The listing builds one solid part. Answer for the finished solid, in the listing's coordinates (mm). A direction names the side the tool comes from. Round coordinates to 2 decimals unless told otherwise and drop trailing zeros. Loops run counter-clockwise (first coordinate to the right, second up) from the corner with the lowest first, then second, coordinate; pieces in that order, holes last. Notation, with made-up numbers: M 58.5,5.5 L 106.5,5.5 A23 ccw 106.5,43.5 Z; hole C 87.25,27.25 d1. An arc over 180 degrees is marked long. Answer as a JSON object with one key per item and string values.
```python
from build123d import *

# Parameters (mm, degrees)
BOSS_EXTRUDE1_DEPTH = 20
SKETCH2_R           = 2.25
SKETCH2_R_2         = 5.25
CUT_EXTRUDE1_DEPTH  = 40


with BuildPart() as part:
    # Sketch1 → Boss-Extrude1 (new, symmetric)
    with BuildSketch(Plane.XY):
        Polygon((-150, 7.75), (-150, -7.75), (150, -7.75), (150, 7.75), (20, 7.75), (20, 0.25), (-20, 0.25), (-20, 7.75), align=None)
    extrude(amount=BOSS_EXTRUDE1_DEPTH, both=True)

    # Sketch2 → Cut-Extrude1 (cut)
    with BuildSketch(Plane(origin=(0, 0.25, 0), x_dir=(1, 0, 0), z_dir=(0, 1, 0))):
        with Locations(Location((15.015, 15, 0), (0, 0, 270))):
            Circle(SKETCH2_R)
        with Locations(Location((-15.015, 15, 0), (0, 0, 180))):
            Circle(SKETCH2_R)
        with Locations(Location((15.015, -15, 0), (0, 0, 180))):
            Circle(SKETCH2_R)
        with Locations(Location((-15.015, -15, 0), (0, 0, 270))):
            Circle(SKETCH2_R)
        with Locations(Location((0, 0, 0), (0, 0, 270))):
            Circle(SKETCH2_R_2)
    extrude(amount=-CUT_EXTRUDE1_DEPTH, mode=Mode.SUBTRACT)


solid = part.part
```
Item 1: The part is cut by section B-B (x = 0). Give the vertices of the cut face in (y, z).
Values follow:
{"outline": "M -7.75,-20 L 0.25,-20 L 0.25,-5.25 L -7.75,-5.25 Z; M -7.75,5.25 L 0.25,5.25 L 0.25,20 L -7.75,20 Z"}
Item 2: Straight lines are drawn through the part: line 1 (X direction, y = -5.75, z = 15.5); line 2 (X direction, y = 1, z = 9.5); line 3 (X direction, y = -3.75, z = -16.5). For each, find the intervals that lie inside material, in ascending order.
Values follow:
{"line 1": "-150 to -17.21, -12.82 to 12.82, 17.21 to 150", "line 2": "-150 to -20, 20 to 150", "line 3": "-150 to -16.69, -13.34 to 13.34, 16.69 to 150"}
Item 3: The part is cut by section A-A (z = 0). Give the vertices of the cut face in (x, y).
Values follow:
{"outline": "M -150,-7.75 L -5.25,-7.75 L -5.25,0.25 L -20,0.25 L -20,7.75 L -150,7.75 Z; M 5.25,-7.75 L 150,-7.75 L 150,7.75 L 20,7.75 L 20,0.25 L 5.25,0.25 Z"}
Item 4: Which of the six approach directions +Z, -Z, +X, -X, +Y, -Y give full straight-line access (tool end or side, diameter ignored) to faces 5 (the face through (86, 7.75, 0)), 6 (the face through (-4, 0.25, -4))?
Values follow:
{"face 5": "+Z, -Z, +X, -X, +Y", "face 6": "+Z, -Z, +Y"}
Item 5: Determine the mould class of faces 1 (the face through (-2, 0, 20)), 2 (the face through (1.6, -3.7, 5)), 3 (the face through (-150, 0, 0)), 4 (the face through (-20, 4, 0)) for opening direction X: released by +X, released by -X, zero draft, split by the parting line, or undercut.
Values follow:
{"face 1": "zero draft", "face 2": "undercut", "face 3": "released by -X", "face 4": "undercut"}
